Print and shaded views of the part. All mm, measured from the part's lowest x, y and z. A direction names the side the tool comes from. Round coordinates to 2 decimals unless told otherwise and drop trailing zeros. Loops run counter-clockwise (first coordinate to the right, second up) from the corner with the lowest first, then second, coordinate; pieces in that order, holes last. Notation, with made-up numbers: M 51,89 L 106,89 A27 cw 106,112 Z; hole C 76.5,28.5 d7. An arc over 180 degrees is marked long. One line per item, written item: value. Start each with the question number.
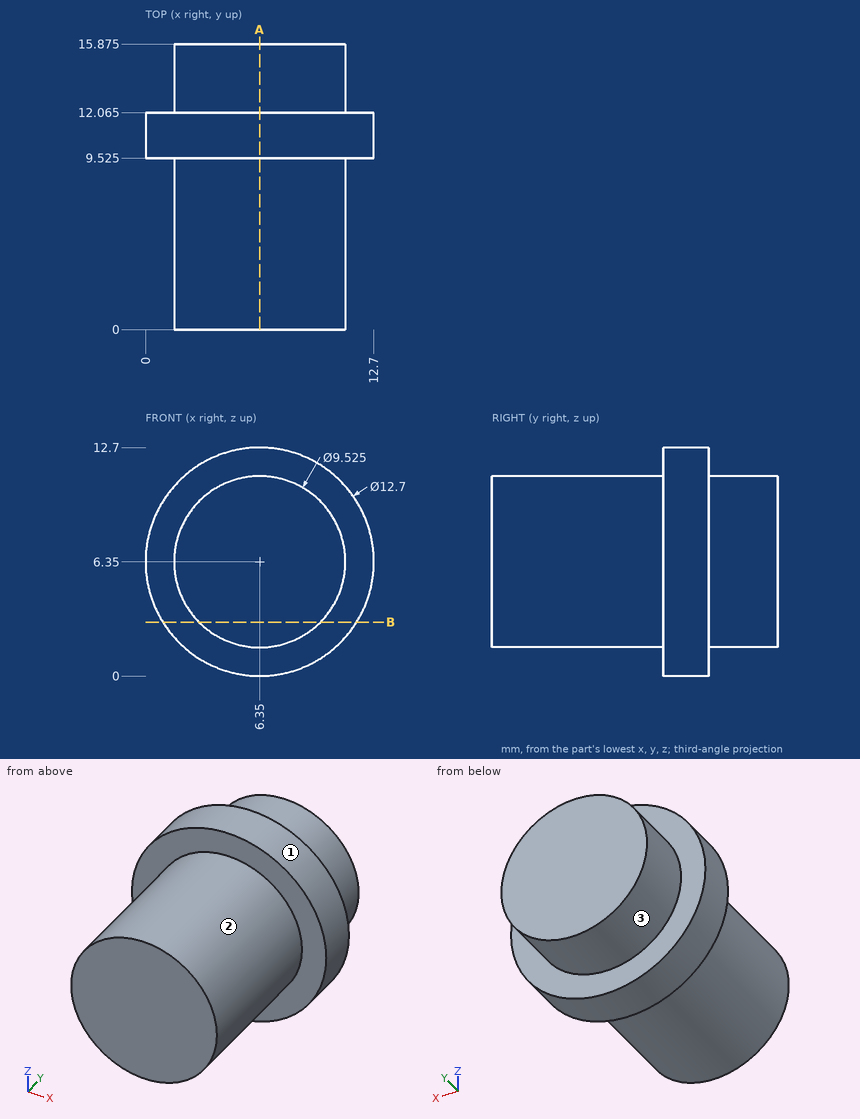
(1) Which spindle directions (+Z, -Z, +X, -X, +Y, -Y) get a long thin tool onto all of the face, cutting with end or side? Do the marked faces 1, 2 and 3. Say none if no direction does.
(2) Flat gauge pins, fed straight in: P1, Ø1, axis at y = 9.5, z = 6.5, coming from the -X side; P2, Ø4, axis at x = 9.5, y = 9.5, coming from the -Z side; P3, Ø2, axis at x = 8, y = 5.5, coming from the -Z side; P4, Ø3, axis at y = 10.5, z = 8, coming from the +X side. Where does each tip first touch, or does it go through?
(3) Slice it at A-A, the plane x = 6.35. List the corners of the cut face in (y, z) (1 decimal), and give its area (3 significant figures).
(4) Probe L1, parallel to Y at x = 11.25, z = 3 (3 decimals); L2, parallel to Z at x = 6.5, y = 12; L3, parallel to Z at x = 10, y = 10.5. List the from-to ranges inside material, lowest first.
(5) Slice it at B-B, the plane z = 3. List the corners of the cut face in (x, y) (3 decimals).
Check result:
1. face 1: +Y, -Y
1. face 2: -Y
1. face 3: +Y
2. P1: stops at x = 0
2. P2: stops at z = 0.11
2. P3: stops at z = 1.63
2. P4: stops at x = 12.7
3. outline: M 0,1.6 L 9.5,1.6 L 9.5,0 L 12.1,0 L 12.1,1.6 L 15.9,1.6 L 15.9,11.1 L 12.1,11.1 L 12.1,12.7 L 9.5,12.7 L 9.5,11.1 L 0,11.1 Z
3. area: 159 mm^2
4. L1: y = 9.525 to 12.065
4. L2: z = 0 to 12.7
4. L3: z = 1.15 to 11.55
5. outline: M 0.956,9.525 L 2.965,9.525 L 2.965,0 L 9.735,0 L 9.735,9.525 L 11.744,9.525 L 11.744,12.065 L 9.735,12.065 L 9.735,15.875 L 2.965,15.875 L 2.965,12.065 L 0.956,12.065 Z
